Here's how the part is built. I have some questions about the finished solid (model axes, mm). A direction names the side the tool comes from. Give positions to 0.01 mm unless a question says otherwise; leave off trailing zeros. Write each loop counter-clockwise with the first axis right and the second up, starting at its lowest first coordinate (ties: lowest second). Pieces come first, ordered by that corner, then holes. Notation, with made-up numbers: (3, 17) - (40, 17) arc R18 cw to (40, 37) - close; hole circle Ø11 at (83.25, 45.5). An arc over 180 degrees is marked (long way). Use a Markdown table: item, result.
```python
from build123d import *

# Parameters (mm, degrees)
SKETCH_1_W          = 7.8
SKETCH_1_H          = 7.8
EXTRUDE_1_DEPTH     = 9.6
SKETCH_6_W          = 6.2
SKETCH_6_H          = 6.2
CUT_EXTRUDE_8_DEPTH = 7.6
SKETCH_9_R          = 2.5
CUT_EXTRUDE_9_DEPTH = 1.8


with BuildPart() as part:
    # Эскиз1 → Бобышка-Вытянуть1 (new body)
    with BuildSketch(Plane.XY):
        Rectangle(SKETCH_1_W, SKETCH_1_H)
    extrude(amount=EXTRUDE_1_DEPTH)

    # Эскиз6 → Вырез-Вытянуть8 (cut)
    with BuildSketch(Plane.XY.offset(9.6)):
        with Locations((-0.8, -0.8)):
            Rectangle(SKETCH_6_W, SKETCH_6_H)
    extrude(amount=-CUT_EXTRUDE_8_DEPTH, mode=Mode.SUBTRACT)

    # Эскиз9 → Вырез-Вытянуть9 (cut)
    with BuildSketch(Plane(origin=(0, 0, 0), x_dir=(-1, 0, 0), z_dir=(0, 0, -1))):
        Circle(SKETCH_9_R)
    extrude(amount=-CUT_EXTRUDE_9_DEPTH, mode=Mode.SUBTRACT)


solid = part.part
```
Item 1: If we section it at B-B, the plane z = 1.5: Write out the boundary of the cut face in (x, y).
Values:
| item | result |
|---|---|
| outline | (-3.9, -3.9) - (3.9, -3.9) - (3.9, 3.9) - (-3.9, 3.9) - close; hole circle Ø5 at (0, 0) |
Item 2: Thinking about a two-plate mould opening in Y: for faces 1 (the cylindrical face through (0.54, -2.44, 0.89)), 2 (the flat face through (-1, 2.3, 6)), 3 (the flat face through (2.3, -1, 6)), which applies, +Y half, -Y half, draft (parallel to the pull), parting line (faces both ways), or undercut?
Values:
| item | result |
|---|---|
| face 1 | undercut |
| face 2 | -Y half |
| face 3 | draft |
Item 3: I need wall thicknesses on line 1 along Y through (x, z) = (0, 0.6); line 2 along Y through (x, z) = (-2.75, 2.5); line 3 along Z through (x, y) = (-1.5, 0.25). Which ranges of each line are inside material? Lowest first, please. Write a range as [from, to].
Values:
| item | result |
|---|---|
| line 1 | y = [-3.9, -2.5], [2.5, 3.9] |
| line 2 | y = [2.3, 3.9] |
| line 3 | z = [1.8, 2] |
Item 4: Will these pins go through, and if not, where does the flat tip stop? pin 1 Ø1 at (x, z) = (-3, 7) entering from -Y; pin 2 Ø2 at (y, z) = (0.5, 8) entering from -X; pin 3 Ø4.5 at (x, y) = (0, 0) entering from +Z.
Values:
| item | result |
|---|---|
| pin 1 | stops at y = 2.3 |
| pin 2 | stops at x = 2.3 |
| pin 3 | stops at z = 2 |
Item 5: If we section it at D-D, the plane z = 4.25: Write out the boundary of the cut face in (x, y), plus the area to 3 significant figures.
Values:
| item | result |
|---|---|
| outline | (-3.9, 2.3) - (2.3, 2.3) - (2.3, -3.9) - (3.9, -3.9) - (3.9, 3.9) - (-3.9, 3.9) - close |
| area | 22.4 mm2 |
Item 6: If we section it at A-A, the plane y = -1.5: Write out the boundary of the cut face in (x, z).
Values:
| item | result |
|---|---|
| outline | (-3.9, 0) - (-2, 0) - (-2, 1.8) - (2, 1.8) - (2, 0) - (3.9, 0) - (3.9, 9.6) - (2.3, 9.6) - (2.3, 2) - (-3.9, 2) - close |
Item 7: For faces 4 (the flat face through (0, 0, 1.8)), 5 (the flat face through (-3.9, 3, 3)), 6 (the flat face through (-1, -1, 2)), which set-ups out of +Z, -Z, +X, -X, +Y, -Y let a thin tool reach every point of the face, with its end or its side?
Values:
| item | result |
|---|---|
| face 4 | -Z |
| face 5 | +Z, -Z, -X, +Y, -Y |
| face 6 | +Z, -X, -Y |
